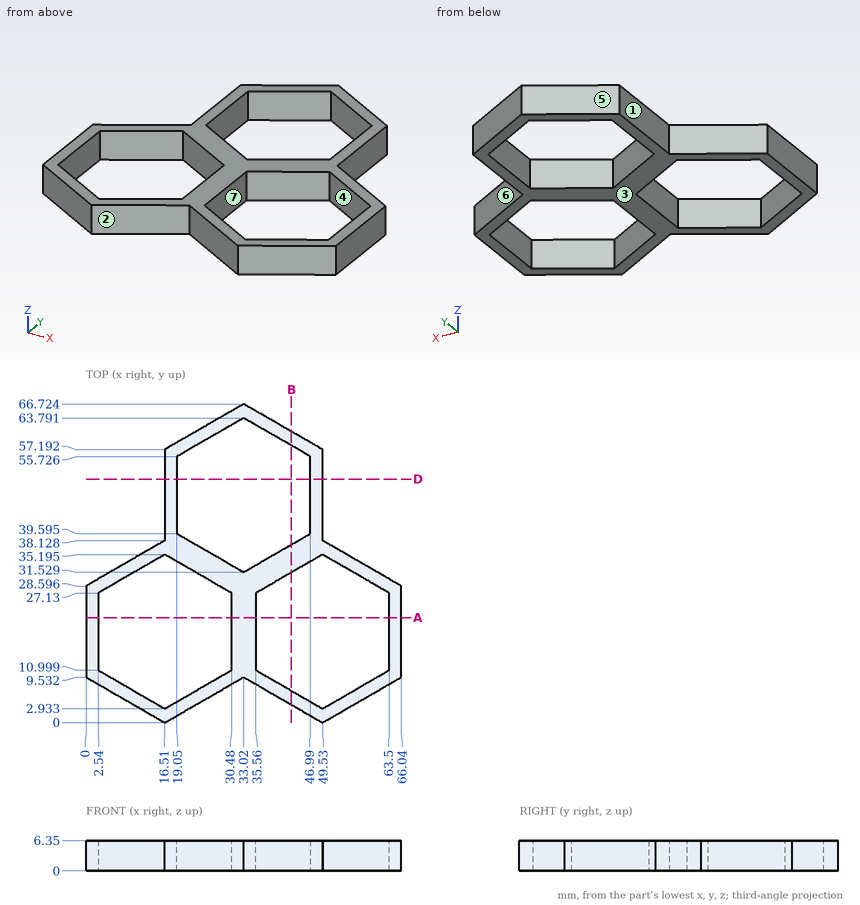
Geometry: see drawing. Coordinates: mm, zero at the bounding-box minimum. A direction names the side the tool comes from. Give positions to 0.01 mm unless a question says otherwise; leave off trailing zeros. Loops run counter-clockwise (first coordinate to the right, second up) from the corner with the lowest first, then second, coordinate; pieces in that order, holes last. Notation, with made-up numbers: M 6.5,71.5 L 57.5,71.5 A29 cw 57.5,99.5 Z; hole C 30,-25 d8. An arc over 180 degrees is marked long. Answer as CSV lines item,"result". Start each with the question number.
1. Pin query (flat end, axial travel): P1, Ø1.9, axis at y = 50, z = 4, coming from the +X side; P2, Ø1.9, axis at y = 48, z = 2, coming from the -X side; P3, Ø1, axis at x = 34, z = 3.5, coming from the +Y side. Return the tip coordinate at first contact, or that it passes through.
2. Pull-direction query (X, two-part tool) for the marked faces 5, 6 and 7; classes: released by +X, released by -X, zero draft, split by the parting line, or undercut.
3. Section B-B on x = 43. State how many separate pieces and enclosed holes the cut face has.
4. Section A-A on y = 22. Return loops of the section in (x, z).
5. Reachability of the marked faces 1, 2, 3 and 4 from +Z, -Z, +X, -X, +Y, -Y: full face, straight path, thin tool, end or side. Return the list, or none.
6. Section D-D on y = 51. Return loops of the section in (x, z).
7. Line query: L1, parallel to X at y = 22.5, z = 5.75; L2, parallel to X at y = 55.5, z = 1; L3, parallel to Y at x = 33, z = 2.5. Output: solid intervals per line, ascending.
Computed values:
1,P1,"stops at x = 49.53"
1,P2,"stops at x = 16.51"
1,P3,"stops at y = 66.45"
2,face 5,"released by -X"
2,face 6,"released by +X"
2,face 7,"undercut"
3,separate pieces,"3"
3,enclosed holes,"0"
4,outline,"M 0,0 L 2.54,0 L 2.54,6.35 L 0,6.35 Z; M 30.48,0 L 35.56,0 L 35.56,6.35 L 30.48,6.35 Z; M 63.5,0 L 66.04,0 L 66.04,6.35 L 63.5,6.35 Z"
5,face 1,"+Z, -Z, -X, +Y"
5,face 2,"+Z, -Z, -Y"
5,face 3,"-Z, +X, -X, +Y, -Y"
5,face 4,"+Z, -Z"
6,outline,"M 16.51,0 L 19.05,0 L 19.05,6.35 L 16.51,6.35 Z; M 46.99,0 L 49.53,0 L 49.53,6.35 L 46.99,6.35 Z"
7,L1,"x = 0 to 2.54, 30.48 to 35.56, 63.5 to 66.04"
7,L2,"x = 16.51 to 19.05, 46.99 to 49.53"
7,L3,"y = 9.52 to 31.54, 63.78 to 66.71"
